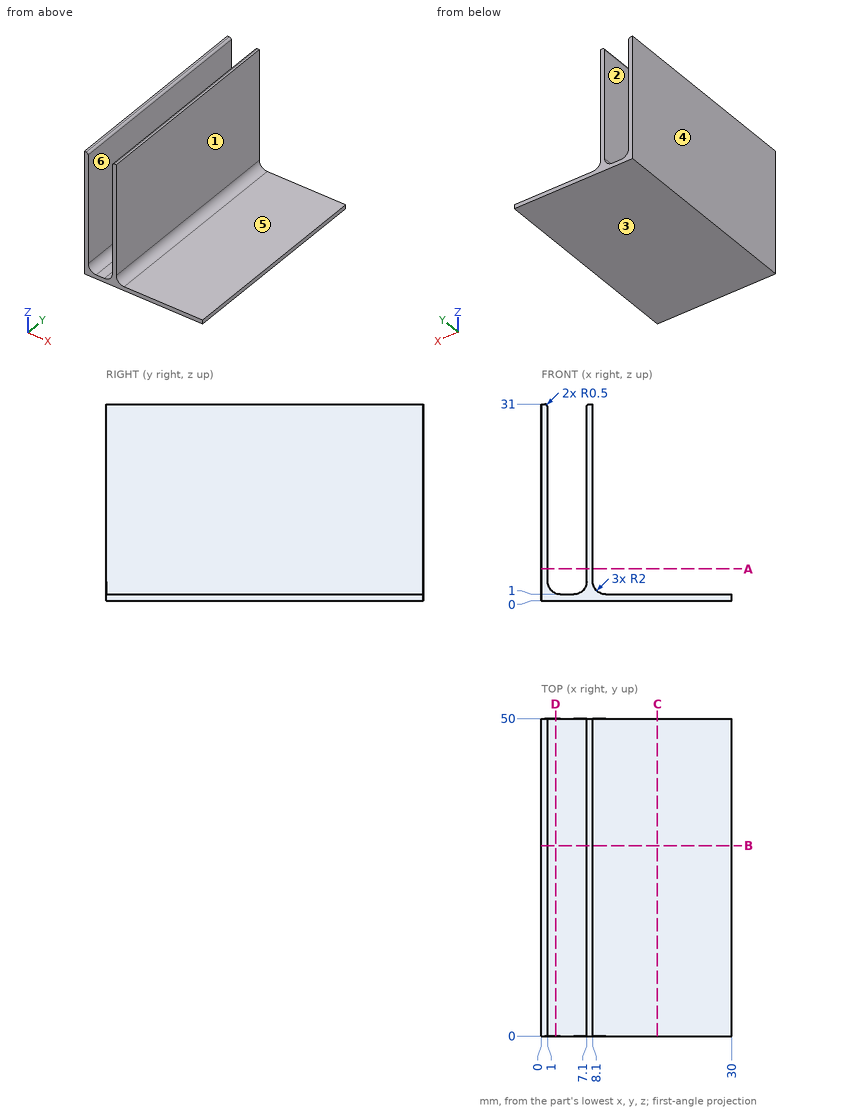
Job drawing, mm, ordinate dimensions from the low corner. One solid piece. A direction names the side the tool comes from. Round coordinates to 2 decimals unless told otherwise and drop trailing zeros. Order: outer loops, then holes, each group sorted by start corner. A loop starts at its lowest first (then second) coordinate and runs counter-clockwise, first axis right, second up. Notation, with made-up numbers: (40.5, 2) -> (53.5, 2) arc R22 ccw to (53.5, 40) -> close; hole circle Ø8 at (38, 48.25). An arc over 180 degrees is marked (long way). Answer in a Markdown table with one row per item.
1) Band-saw the part on D-D on x = 2.25. Give the cut face in (y, z).
Values:
| item | result |
|---|---|
| outline | (0, 0) -> (50, 0) -> (50, 1.15) -> (0, 1.15) -> close |
2) Mould opens along X. For the marked faces 1, 2 and 3 say: released by +X, released by -X, zero draft, split by the parting line, or undercut.
Values:
| item | result |
|---|---|
| face 1 | released by +X |
| face 2 | undercut |
| face 3 | zero draft |
3) Band-saw the part on C-C on x = 18.25. Give the cut face in (y, z), and give its area (3 significant figures).
Values:
| item | result |
|---|---|
| outline | (0, 0) -> (50, 0) -> (50, 1) -> (0, 1) -> close |
| area | 50.0 mm2 |
4) Which spindle directions (+Z, -Z, +X, -X, +Y, -Y) get a long thin tool onto all of the face, cutting with end or side? Do the marked faces 4, 5 and 6. Say none if no direction does.
Values:
| item | result |
|---|---|
| face 4 | +Z, -Z, -X, +Y, -Y |
| face 5 | +Z, +X, +Y, -Y |
| face 6 | +Z, +Y, -Y |
5) Band-saw the part on A-A on z = 5. Give the cut face in (x, y), and give its area (3 significant figures).
Values:
| item | result |
|---|---|
| outline | (0, 0) -> (1, 0) -> (1, 50) -> (0, 50) -> close; (7.1, 0) -> (8.1, 0) -> (8.1, 50) -> (7.1, 50) -> close |
| area | 100 mm2 |
6) Band-saw the part on B-B on y = 30. Give the cut face in (x, z), and give its area (3 significant figures).
Values:
| item | result |
|---|---|
| outline | (0, 0) -> (30, 0) -> (30, 1) -> (10.1, 1) arc R2 cw to (8.1, 3) -> (8.1, 31) -> (7.6, 31) arc R0.5 ccw to (7.1, 30.5) -> (7.1, 3) arc R2 cw to (5.1, 1) -> (3, 1) arc R2 cw to (1, 3) -> (1, 30.5) arc R0.5 ccw to (0.5, 31) -> (0, 31) -> close |
| area | 92.5 mm2 |
7) Wall check: L1, parallel to X at y = 36.5, z = 5.5; L2, parallel to Z at x = 27.5, y = 3; L3, parallel to Z at x = 7.25, y = 36. Give the ranges that are in metal, low to high.
Values:
| item | result |
|---|---|
| L1 | 0 to 1, 7.1 to 8.1 |
| L2 | 0 to 1 |
| L3 | 0 to 30.86 |
8) Pin check, flat tips, straight feed: P1, Ø8, axis at y = 24, z = 19, coming from the +X side; P2, Ø5, axis at x = 4, z = 23.5, coming from the -Y side; P3, Ø10, axis at x = 24.5, y = 19.5, coming from the +Z side. Stop position of each tip, or through.
Values:
| item | result |
|---|---|
| P1 | x = 8.1 |
| P2 | through |
| P3 | z = 1 |
